Can you work these out from the model? Positions are in its coordinate system, mm. Coordinates: 2 decimals unless noted, no trailing zeros. Order: outer loops, then holes, each group sorted by start corner. A loop starts at its lowest first (then second) coordinate and runs counter-clockwise, first axis right, second up. Notation, with made-up numbers: (87, 34.25) -> (132, 34.25) arc R17 ccw to (132, 63.25) -> close; hole circle Ø9 at (66, 21.25). An arc over 180 degrees is marked (long way). Use a Markdown table: item, result. Add a question column.
1. If I drill on line 1 along X through (y, z) = (5.25, -104.5); line 2 along X through (y, z) = (3.5, -133.5), over which ranges is the centre line in solid material (lowest first)? Write a range as from..to.
2. Suppose I cut it at A-A, the plane y = 2.25. List the corners of the cut face in (x, z) for me, then the cut area to 3 significant figures.
3. Suppose I cut it at B-B, the plane x = -3. List the corners of the cut face in (y, z) for me, then the cut area to 3 significant figures.
4. Suppose I cut it at C-C, the plane z = -22.5. List the corners of the cut face in (x, y) for me, then the cut area to 3 significant figures.
5. For pin 1 Ø1.5 at (x, y) = (117, 4.5) entering from -Z; pin 2 Ø4 at (x, z) = (-49.5, 21.5) entering from -Y; pin 3 Ø5 at (x, y) = (49.5, 6) entering from -Z; pin 4 Ø1 at (y, z) = (3, 40.5) entering from -X, each with a flat end and sliding along its axis, tell me the tip position at first contact or that it passes through.
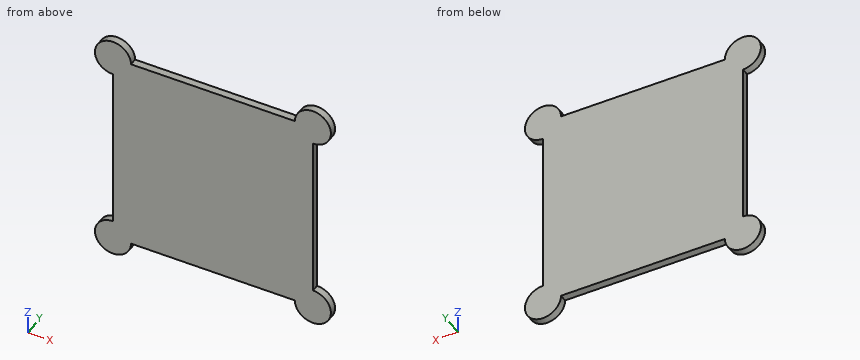
```python
from build123d import *

# Parameters (mm, degrees)
SKETCH_1_R      = 24
SKETCH_1_W      = 266
SKETCH_1_H      = 266
EXTRUDE_1_DEPTH = 10


with BuildPart() as part:
    # 草图1 → 凸台-拉伸1 (new body)
    with BuildSketch(Plane(origin=(0, 0, 0), x_dir=(1, 0, 0), z_dir=(0, 1, 0))):
        with BuildLine():
            Line((-133, 109), (-133, 133))
            Line((-133, 133), (-109, 133))
            ThreePointArc((-109, 133), (-149.970562748, 149.970562748), (-133, 109))
        make_face()
        with BuildLine():
            Line((-109, 133), (-133, 133))
            Line((-133, 133), (-133, 109))
            ThreePointArc((-133, 109), (-116.029437252, 116.029437252), (-109, 133))
        make_face()
        with Locations((-133, -133)):
            Circle(SKETCH_1_R)
        with Locations((133, -133)):
            Circle(SKETCH_1_R)
        with Locations((133, 133)):
            Circle(SKETCH_1_R)
        with Locations((-133, 133)):
            Circle(SKETCH_1_R)
        Rectangle(SKETCH_1_W, SKETCH_1_H)
        with BuildLine():
            ThreePointArc((157, 133), (133, 157), (109, 133))
            Line((109, 133), (133, 133))
            Line((133, 133), (133, 109))
            ThreePointArc((133, 109), (149.970562748, 116.029437252), (157, 133))
        make_face()
        with BuildLine():
            Line((133, 133), (109, 133))
            ThreePointArc((109, 133), (116.029437252, 116.029437252), (133, 109))
            Line((133, 109), (133, 133))
        make_face()
        with BuildLine():
            ThreePointArc((157, -133), (149.970562748, -116.029437252), (133, -109))
            Line((133, -109), (133, -133))
            Line((133, -133), (109, -133))
            ThreePointArc((109, -133), (133, -157), (157, -133))
        make_face()
        with BuildLine():
            Line((133, -133), (133, -109))
            ThreePointArc((133, -109), (116.029437252, -116.029437252), (109, -133))
            Line((109, -133), (133, -133))
        make_face()
        with BuildLine():
            ThreePointArc((-109, -133), (-116.029437252, -116.029437252), (-133, -109))
            Line((-133, -109), (-133, -133))
            Line((-133, -133), (-109, -133))
        make_face()
        with BuildLine():
            Line((-133, -133), (-133, -109))
            ThreePointArc((-133, -109), (-149.970562748, -149.970562748), (-109, -133))
            Line((-109, -133), (-133, -133))
        make_face()
    extrude(amount=EXTRUDE_1_DEPTH)


solid = part.part
```
Worked out:
| question | item | result |
|---|---|---|
| 1 | line 1 | x = -133..133 |
| 1 | line 2 | x = -156.99..-109.01, 109.01..156.99 |
| 2 | outline | (-133, -109) arc R24 ccw (long way) to (-109, -133) -> (109, -133) arc R24 ccw (long way) to (133, -109) -> (133, 109) arc R24 ccw (long way) to (109, 133) -> (-109, 133) arc R24 ccw (long way) to (-133, 109) -> close |
| 2 | area | 76,200 mm² |
| 3 | outline | (0, -133) -> (10, -133) -> (10, 133) -> (0, 133) -> close |
| 3 | area | 2,660 mm² |
| 4 | outline | (-133, 0) -> (133, 0) -> (133, 10) -> (-133, 10) -> close |
| 4 | area | 2,660 mm² |
| 5 | pin 1 | stops at z = -151.53 |
| 5 | pin 2 | stops at y = 0 |
| 5 | pin 3 | stops at z = -133 |
| 5 | pin 4 | stops at x = -133 |
